Here's the drawing with two shaded views (mm, measured from the low corner). I have some questions. A direction names the side the tool comes from. Coordinates: 2 decimals unless noted, no trailing zeros. Loops run counter-clockwise (first coordinate to the right, second up) from the corner with the lowest first, then second, coordinate; pieces in that order, holes last.
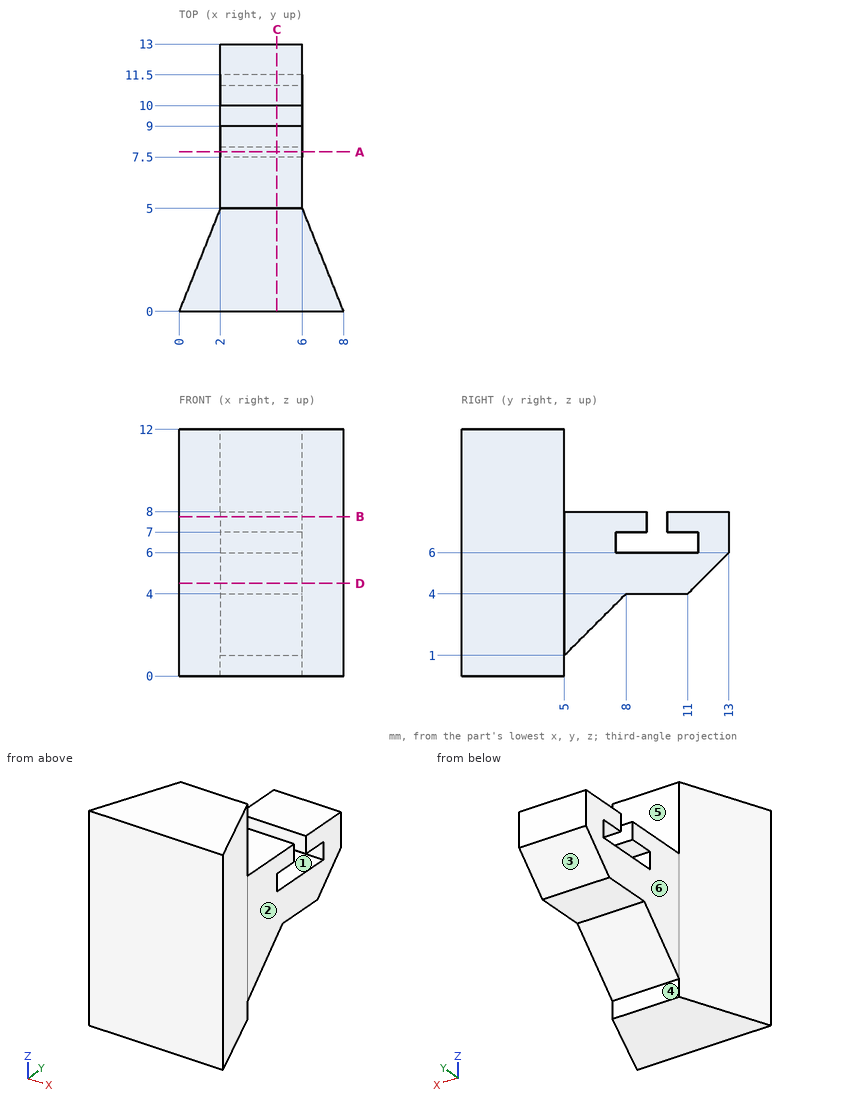
Q1. Will these pins go through, and if not, where does the flat tip stop? P1, Ø4.5, axis at x = 3.5, y = 7.5, coming from the +Z side; P2, Ø0.8, axis at x = 4.5, y = 8.5, coming from the -Z side; P3, Ø6, axis at y = 11, z = 7.5, coming from the -X side.
Q2. Please list where these lines run through material, in increasing order: probe 1 along Z at (x, y) = (5, 8.25); probe 2 along X at (y, z) = (11.25, 5); probe 3 along Y at (x, z) = (3, 9.5).
Q3. Suppose I cut it at B-B on z = 7.75. Write out the boundary of the cut face in (x, y), and give its area (3 significant figures).
Q4. Suppose I cut it at A-A on y = 7.75. Write out the boundary of the cut face in (x, z), and give its area (3 significant figures).
Q5. We'd pull the mould along Z, two halves only. Please class the marked faces 1, 2 and 3: pulls with the +Z half, pulls with the -Z half, needs draft (parallel to the pull), parting line crosses it, or undercut.
Q6. Suppose I cut it at D-D on z = 4.5. Write out the boundary of the cut face in (x, y).
Q7. Suppose I cut it at C-C on x = 4.75. Write out the boundary of the cut face in (y, z).
Q8. For the marked faces 4, 5 and 6, which set-ups out of +Z, -Z, +X, -X, +Y, -Y let a thin tool reach every point of the face, with its end or its side?
Check values:
1. P1: stops at z = 8
1. P2: stops at z = 4
1. P3: stops at x = 2
2. probe 1: z = 4 to 6, 7 to 8
2. probe 2: x = 2 to 6
2. probe 3: y = 0 to 5
3. outline: (0, 0) - (8, 0) - (6, 5) - (6, 9) - (2, 9) - (2, 5) - close; (2, 10) - (6, 10) - (6, 13) - (2, 13) - close
3. area: 58.0 mm2
4. outline: (2, 3.75) - (6, 3.75) - (6, 6) - (2, 6) - close; (2, 7) - (6, 7) - (6, 8) - (2, 8) - close
4. area: 13.0 mm2
5. face 1: undercut
5. face 2: needs draft
5. face 3: pulls with the -Z half
6. outline: (0, 0) - (8, 0) - (6, 5) - (6, 11.5) - (2, 11.5) - (2, 5) - close
7. outline: (0, 0) - (5, 0) - (5, 1) - (8, 4) - (11, 4) - (13, 6) - (13, 8) - (10, 8) - (10, 7) - (11.5, 7) - (11.5, 6) - (7.5, 6) - (7.5, 7) - (9, 7) - (9, 8) - (5, 8) - (5, 12) - (0, 12) - close
8. face 4: -Z, +X, -X, +Y
8. face 5: +Z, +X, -X, +Y
8. face 6: +Z, -Z, -X, +Y
